Geometry: final body of the model. Coordinates: model frame, mm. Round coordinates to 2 decimals unless told otherwise and drop trailing zeros. Loops run counter-clockwise (first coordinate to the right, second up) from the corner with the lowest first, then second, coordinate; pieces in that order, holes last. Notation, with made-up numbers: M -16,16 L -9,16 A11 cw -9,31 Z; hole C -39.75,83.25 d2. An arc over 180 degrees is marked long. Answer as a JSON object with one key per item and string values.
Autodesk Inventor part; units mm, degrees
ref_plane "YZ Plane" through (0, 0, 0) normal (1, 0, 0) x (0, 1, 0)
ref_plane "XZ Plane" through (0, 0, 0) normal (0, 1, 0) x (-1, 0, 0)
ref_plane "XY Plane" through (0, 0, 0) normal (0, 0, 1) x (1, 0, 0)
sketch "スケッチ1" plane through (0, 0, 0) normal (1, 0, 0) x (0, 1, 0)
  line L0 (0, 0) -> (147.3717, -500)
  arc A0 (0, 0) -> (37.8967, -343.7392) centre (1577.8776, 0) ccw
  arc A1 (37.8967, -343.7392) -> (147.3717, -500) centre (281.8923, -289.2769) ccw
  arc A2 (0, 0) -> (-50, -259.8835) centre (293.1864, -191.1589) ccw
  arc A3 (-50, -259.8835) -> (147.3717, -500) centre (273.5758, -195.086) ccw
  line L1 (0, -630.6128) -> (0, 110.8282)
  point P0 (35.1596, -247.5153)
  dimension "d1" = 500
  dimension "d2" = 250
  dimension "d3" = 1577.8776
  dimension "d4" = 250
  dimension "d6" = 350
  dimension "d21" = 330
  dimension "d26" = 50
extrude "押し出し1" add sketch "スケッチ1" along normal mid plane 50 contours L1 A3 A2 | A0 A1 A3 L1
fillet "フィレット1" radius 10 1 edges at (0, 0, 0)
fillet "フィレット1" radius 5 1 edges at (0, 147.3717, -500)
sketch "スケッチ2" plane through (25, 0, 0) normal (1, 0, 0) x (0, 0, -1)
  circle A0 centre (96.4602, -19.5814) radius 7.5
  circle A1 centre (376.4602, 20.4186) radius 7.5
  arc A2 (36.2306, 0.416) -> (31.9103, -18.4863) centre (36.4602, -9.5814) ccw
  point P0 (0, 0)
  dimension "d11" = 15
  dimension "d12" = 15
  dimension "d13" = 280
  dimension "d16" = 40
  dimension "d24" = 60
  dimension "d25" = 10
extrude "押し出し2" cut sketch "スケッチ2" against normal through all
properties part number "styro_50_main" material "ポリスチレン、耐衝撃性"
1) Pull-direction query (Z, two-part tool) for faces 1 (the cylindrical face through (-0.35, 4.49, -386.12)), 2 (the cylindrical face through (0.35, 17.55, -383.39)), 3 (the cylindrical face through (-0.35, 64.444, -412.631)), 4 (the flat face through (-25, -5, -251)); classes: +Z half, -Z half, draft (parallel to the pull), parting line (faces both ways), or undercut.
Results:
{"face 1": "-Z half", "face 2": "undercut", "face 3": "+Z half", "face 4": "draft"}
2) Section query A-A (z = -64). Return the cut outline in (x, y).
Results:
{"outline": "M -25,-32.9 L 25,-32.9 L 25,1.3 L -25,1.3 Z"}
3) Ray query, line 1 (Z direction, x = -15.5, y = -21); line 2 (Y direction, x = -15, z = -382); line 3 (Y direction, x = 18, z = -93). Return the intervals inside material, ascending.
Results:
{"line 1": "-343.83 to -103.82, -89.1 to -36.93", "line 2": "1.61 to 15.36, 25.47 to 49.72", "line 3": "-42.77 to -26.24, -12.93 to 2.74"}
4) Pin query (flat end, axial travel): P1, Ø2, axis at x = 13, y = -7, coming from the +Z side; P2, Ø4, axis at y = 35.5, z = -321, coming from the +X side; P3, Ø6, axis at x = -17.5, z = -412, coming from the +Y side; P4, Ø6, axis at x = 1, z = -113, coming from the -Y side. Return the tip coordinate at first contact, or that it passes through.
Results:
{"P1": "z = -26.59", "P2": "through", "P3": "y = 65.81", "P4": "y = -48.65"}
5) Section query C-C (x = -8). Count the separate pieces of the cut face and the enclosed holes in it, and give its area (3 significant figures).
Results:
{"separate pieces": "1", "enclosed holes": "2", "area": "23,200 mm2"}
6) Section query B-B (y = 59.5). Return the cut outline in (x, z), and give its area (3 significant figures).
Results:
{"outline": "M -25,-446.23 L 25,-446.23 L 25,-403.48 L -25,-403.48 Z", "area": "2,140 mm2"}
